For this review, take the finished solid that the model builds, in its own axes (mm). Face numbers are marked on the shaded views. A direction names the side the tool comes from. Give positions to 0.01 mm unless a question says otherwise; leave off trailing zeros. Write each loop counter-clockwise with the first axis right and the second up, starting at its lowest first coordinate (ties: lowest second). Pieces come first, ordered by that corner, then holes. Notation, with made-up numbers: M -21,-32 L 35,-32 A28 cw 35,-8 Z; hole C 23.25,-30 d6. An arc over 180 degrees is marked long. Use one line per item in the form item = value. Start each with the question number.
Q1. For probe 1 along Z at (x, y) = (0, 27); probe 2 along X at (y, z) = (7, 7.25), list the stretches that pass through material, from the lowest coordinate up. Write a range as [from, to].
Q2. Tool access review of the marked faces 5, 6 and 7: name each direction out of +Z, -Z, +X, -X, +Y, -Y from which nothing blocks a thin tool from reaching the whole face with its end or side.
Q3. Consider section A-A on x = 0. Write out the cut boundary in (y, z), and give its area (3 significant figures).
Q4. Consider section B-B on z = 1.5. Write out the cut boundary in (x, y), and give its area (3 significant figures).
Q5. Clearance check with flat-ended pins moving along their axes: pin 1 Ø1.7 at (x, y) = (1, 28.5) entering from +Z; pin 2 Ø1 at (y, z) = (7.5, -2.5) entering from -X. State where each tip first meets the part, or that it passes through.
Q6. Mouldability with a two-part tool opening along X and no side actions: class the marked faces 1, 2, 3 and 4 as released by +X, released by -X, zero draft, split by the parting line, or undercut.
Q7. Consider section C-C on x = 5. Write out the cut boundary in (y, z), and give its area (3 significant figures).
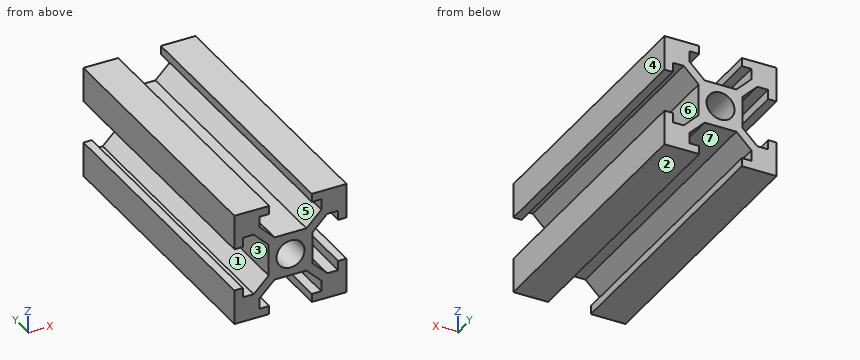
```python
from build123d import *

# Parameters (mm, degrees)
SKETCH_1_W      = 1.5
SKETCH_1_H      = 1.7
SKETCH_1_W_2    = 1.7
SKETCH_1_H_2    = 1.5
SKETCH_1_W_3    = 7.8
SKETCH_1_H_3    = 7.8
SKETCH_1_R      = 2.5
EXTRUDE_1_DEPTH = 50


with BuildPart() as part:
    # 草图1 → 凸台-拉伸1 (new body)
    with BuildSketch(Plane(origin=(0, 0, 0), x_dir=(1, 0, 0), z_dir=(0, 1, 0))):
        Polygon((5.5, 8.5), (5.5, 6.560660172), (5.5, 5.5), (6.560660172, 5.5), (8.5, 5.5), (10, 5.5), (10, 10), (5.5, 10), align=None)
        with Locations((9.25, 4.65)):
            Rectangle(SKETCH_1_W, SKETCH_1_H)
        Polygon((5.5, 6.560660172), (2.839339828, 3.9), (3.9, 3.9), (3.9, 2.839339828), (6.560660172, 5.5), (5.5, 5.5), align=None)
        with Locations((4.65, 9.25)):
            Rectangle(SKETCH_1_W_2, SKETCH_1_H_2)
        Rectangle(SKETCH_1_W_3, SKETCH_1_H_3)
        Circle(SKETCH_1_R, mode=Mode.SUBTRACT)
        with Locations((-4.65, 9.25)):
            Rectangle(SKETCH_1_W_2, SKETCH_1_H_2)
        Polygon((-8.5, 5.5), (-6.560660172, 5.5), (-5.5, 5.5), (-5.5, 6.560660172), (-5.5, 8.5), (-5.5, 10), (-10, 10), (-10, 5.5), align=None)
        with Locations((-9.25, 4.65)):
            Rectangle(SKETCH_1_W, SKETCH_1_H)
        Polygon((-5.5, 5.5), (-6.560660172, 5.5), (-3.9, 2.839339828), (-3.9, 3.9), (-2.839339828, 3.9), (-5.5, 6.560660172), align=None)
        Polygon((-5.5, -5.5), (-6.560660172, -5.5), (-8.5, -5.5), (-10, -5.5), (-10, -10), (-5.5, -10), (-5.5, -8.5), (-5.5, -6.560660172), align=None)
        with Locations((-4.65, -9.25)):
            Rectangle(SKETCH_1_W_2, SKETCH_1_H_2)
        with Locations((-9.25, -4.65)):
            Rectangle(SKETCH_1_W, SKETCH_1_H)
        Polygon((-3.9, -3.9), (-3.9, -2.839339828), (-6.560660172, -5.5), (-5.5, -5.5), (-5.5, -6.560660172), (-2.839339828, -3.9), align=None)
        Polygon((3.9, -3.9), (2.839339828, -3.9), (5.5, -6.560660172), (5.5, -5.5), (6.560660172, -5.5), (3.9, -2.839339828), align=None)
        Polygon((5.5, -5.5), (5.5, -6.560660172), (5.5, -8.5), (5.5, -10), (10, -10), (10, -5.5), (8.5, -5.5), (6.560660172, -5.5), align=None)
        with Locations((9.25, -4.65)):
            Rectangle(SKETCH_1_W, SKETCH_1_H)
        with Locations((4.65, -9.25)):
            Rectangle(SKETCH_1_W_2, SKETCH_1_H_2)
    extrude(amount=EXTRUDE_1_DEPTH)


solid = part.part
```
Working result:
q1.probe_1 = [-3.9, -2.5], [2.5, 3.9]
q1.probe_2 = [-10, -5.5], [5.5, 10]
q2.face_5 = +Y, -Y
q2.face_6 = +X, +Y, -Y
q2.face_7 = -Z, +Y, -Y
q3.outline = M 0,-3.9 L 50,-3.9 L 50,-2.5 L 0,-2.5 Z; M 0,2.5 L 50,2.5 L 50,3.9 L 0,3.9 Z
q3.area = 140 mm²
q4.outline = M -3.9,0 L -2,0 L -2,50 L -3.9,50 Z; M 2,0 L 3.9,0 L 3.9,50 L 2,50 Z
q4.area = 190 mm²
q5.pin_1 = 3.9
q5.pin_2 = -4.06
q6.face_1 = undercut
q6.face_2 = zero draft
q6.face_3 = released by -X
q6.face_4 = released by +X
q7.outline = M 0,-10 L 50,-10 L 50,-8.5 L 0,-8.5 Z; M 0,-6.06 L 50,-6.06 L 50,-3.94 L 0,-3.94 Z; M 0,3.94 L 50,3.94 L 50,6.06 L 0,6.06 Z; M 0,8.5 L 50,8.5 L 50,10 L 0,10 Z
q7.area = 362 mm²
